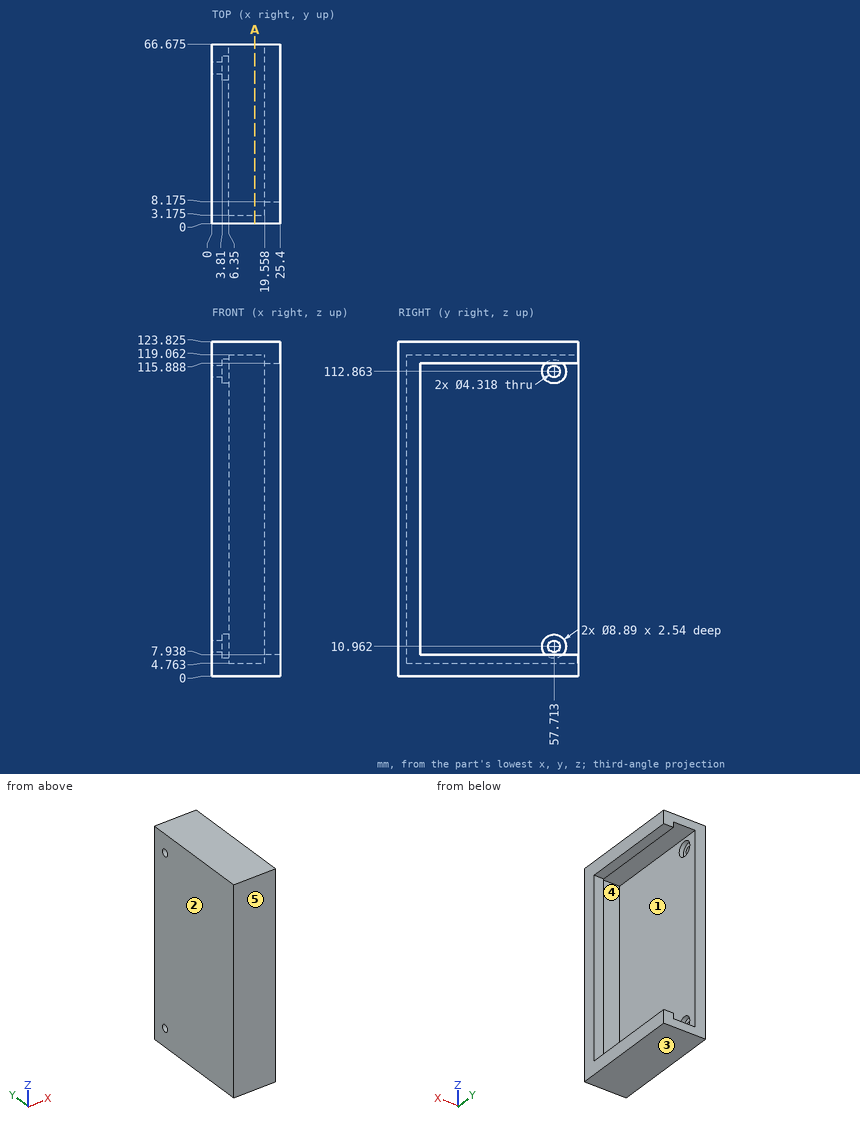
Answer from the drawing. Dimensions are ordinates in mm from the lowest x, y and z of the part. A direction names the side the tool comes from. Give positions to 0.01 mm unless a question says otherwise; leave off trailing zeros. Order: outer loops, then holes, each group sorted by start corner. A loop starts at its lowest first (then second) coordinate and runs counter-clockwise, first axis right, second up.
(1) For a pull along Z with two mould halves and no side action, classify the marked faces 1, 2 and 3 as released by +Z, released by -Z, zero draft, split by the parting line, or undercut.
(2) Given pin 1 (4.5 mm diameter, centred on y = 58, z = 12.5, fed in from +X); pin 2 (3 mm diameter, centred on x = 22, z = 84.5, fed in from +Y) (1 decimal); pin 3 (6 mm diameter, centred on y = 39, z = 23, fed in from +X), each flat-ended and moving along its own axis, determine where each tip first touches the part or whether it passes through.
(3) Straight lines are drawn through the part: L1, parallel to X at y = 6, z = 62.5; L2, parallel to Z at x = 8, y = 26 (1 decimal); L3, parallel to Z at x = 20.75, y = 14 (1 decimal). For each, find the intervals that lie inside material, in ascending order.
(4) Find section A-A (x = 16). Give the vertices of the cut face in (y, z) (1 decimal).
(5) For the marked faces 4 and 5, determine the directions among +Z, -Z, +X, -X, +Y, -Y from which every point of the face is accessible in a straight line to the end or side of a thin tool.
Result sheet:
1. face 1: undercut
1. face 2: zero draft
1. face 3: released by -Z
2. pin 1: stops at x = 3.81
2. pin 2: stops at y = 8.2
2. pin 3: stops at x = 6.35
3. L1: x = 0 to 6.35, 19.56 to 25.4
3. L2: z = 0 to 4.8, 119.1 to 123.8
3. L3: z = 0 to 7.9, 115.9 to 123.8
4. outline: (0, 0) - (66.7, 0) - (66.7, 4.8) - (3.2, 4.8) - (3.2, 119.1) - (66.7, 119.1) - (66.7, 123.8) - (0, 123.8) - close
5. face 4: +Y
5. face 5: +Z, -Z, +X, -X, -Y
